```python
from build123d import *

# Parameters (mm, degrees)
SKETCH1_W           = 3.175
SKETCH1_H           = 14.816666666
BOSS_EXTRUDE2_DEPTH = 3.175


with BuildPart() as part:
    # Sketch1 → Boss-Extrude2 (new body)
    with BuildSketch(Plane(origin=(0, 0, 0), x_dir=(1, 0, 0), z_dir=(0, 1, 0))):
        Polygon((3.175, 0), (3.175, -14.816666667), (3.175, -29.633333333), (3.175, -44.45), (29.5656, -44.45), (29.5656, -29.633333333), (29.5656, -14.816666667), (29.5656, 0), align=None)
        with Locations((1.5875, -22.225)):
            Rectangle(SKETCH1_W, SKETCH1_H)
        with Locations((31.1531, -22.225)):
            Rectangle(SKETCH1_W, SKETCH1_H)
    extrude(amount=BOSS_EXTRUDE2_DEPTH)


solid = part.part
```
For this review, take the finished solid that the model builds, in its own axes (mm). A direction names the side the tool comes from. Round coordinates to 2 decimals unless told otherwise and drop trailing zeros. Write each loop counter-clockwise with the first axis right and the second up, starting at its lowest first coordinate (ties: lowest second). Pieces come first, ordered by that corner, then holes. Notation, with made-up numbers: (-33, 49) - (-4, 49) arc R19 ccw to (-4, 71) - close; hole circle Ø9 at (12, -24). An arc over 180 degrees is marked (long way). Put each result on its own line as item: value.
Q1. Machinability: for faces 1 (the face through (3.175, 2, 7)), 2 (the face through (16, 0, 22)), 3 (the face through (3.175, 2, 37)), 4 (the face through (31, 2, 29.633)), 5 (the face through (29.566, 2, 8)), which of the approach directions +Z, -Z, +X, -X, +Y, -Y give a long, thin tool a straight path to every point of the face, cutting with its end or side? Answer none if there is none.
Solved:
face 1: -Z, -X, +Y, -Y
face 2: +Z, -Z, +X, -X, -Y
face 3: +Z, -X, +Y, -Y
face 4: +Z, +X, +Y, -Y
face 5: -Z, +X, +Y, -Y
Q2. Insertion check: pin 1 Ø1.6 at (x, y) = (31.5, 2) entering from -Z; pin 2 Ø1.6 at (y, z) = (1, 5.5) entering from -X (3 decimals). Each pin has a flat end and moves straight along its axis. Give the tip position at first contact, or say it passes through.
Solved:
pin 1: stops at z = 14.82
pin 2: stops at x = 3.175
Q3. We need section B-B (z = 9.5). Give the boundary of the cut face in (x, y) (3 decimals), and give its area (3 significant figures).
Solved:
outline: (3.175, 0) - (29.566, 0) - (29.566, 3.175) - (3.175, 3.175) - close
area: 83.8 mm2
Q4. We need section A-A (y = 2.25). Give the boundary of the cut face in (x, z) (3 decimals).
Solved:
outline: (0, 14.817) - (3.175, 14.817) - (3.175, 0) - (29.566, 0) - (29.566, 14.817) - (32.741, 14.817) - (32.741, 29.633) - (29.566, 29.633) - (29.566, 44.45) - (3.175, 44.45) - (3.175, 29.633) - (0, 29.633) - close
Q5. Wall thickness on probe 1 along Z at (x, y) = (30, 2.3); probe 2 along X at (y, z) = (1.95, 8.5) (3 decimals): over which ranges is each line inside the solid? List them lowest first.
Solved:
probe 1: z = 14.82 to 29.63
probe 2: x = 3.175 to 29.566
